Can you work these out from the drawing? Everything is in mm from the part's minimum corner. Round coordinates to 2 decimals unless told otherwise and drop trailing zeros. Loops run counter-clockwise (first coordinate to the right, second up) from the corner with the lowest first, then second, coordinate; pieces in that order, holes last. Notation, with made-up numbers: (71.5, 0.5) -> (120.5, 0.5) arc R30 ccw to (120.5, 22.5) -> close; hole circle Ø8 at (46, 9.25). An arc over 180 degrees is marked (long way). Answer as a JSON object with one key per item and string values.
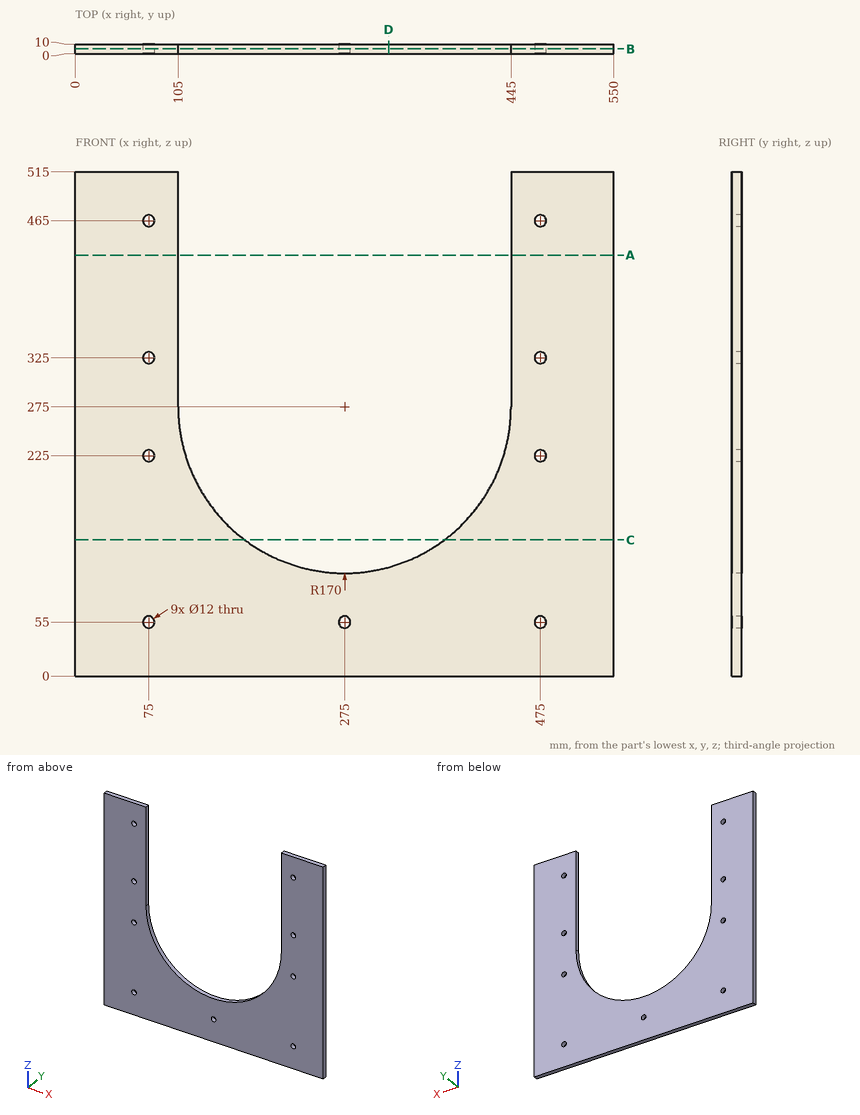
Q1. I want a section at A-A, the plane z = 430. Write out the boundary of the cut face in (x, y), then the cut area to 3 significant figures.
Determined:
{"outline": "(0, 0) -> (105, 0) -> (105, 10) -> (0, 10) -> close; (445, 0) -> (550, 0) -> (550, 10) -> (445, 10) -> close", "area": "2,100 mm²"}
Q2. I want a section at C-C, the plane z = 139. Write out the boundary of the cut face in (x, y).
Determined:
{"outline": "(0, 0) -> (173, 0) -> (173, 10) -> (0, 10) -> close; (377, 0) -> (550, 0) -> (550, 10) -> (377, 10) -> close"}
Q3. I want a section at B-B, the plane y = 5. Give the number of separate pieces and of enclosed holes in the cut face, then the cut area to 3 significant figures.
Determined:
{"separate pieces": "1", "enclosed holes": "9", "area": "155,000 mm²"}
Q4. If I drill on L1, parallel to Z at x = 475, y = 5; L2, parallel to X at y = 5, z = 325; L3, parallel to X at y = 6.75, z = 59, over which ranges is the centre line in solid material (lowest first)? Write a range as [from, to].
Determined:
{"L1": "[0, 49], [61, 219], [231, 319], [331, 459], [471, 515]", "L2": "[0, 69], [81, 105], [445, 469], [481, 550]", "L3": "[0, 70.53], [79.47, 270.53], [279.47, 470.53], [479.47, 550]"}
Q5. I'm going to push flat-ended pins straight in: pin 1 (11 mm diameter, centred on x = 75, z = 325, fed in from -Y); pin 2 (6 mm diameter, centred on x = 263, y = 3, fed in from +Z). Where does each tip first touch, or does it pass through?
Determined:
{"pin 1": "through", "pin 2": "z = 105.66"}
Q6. I want a section at D-D, the plane x = 320. Write out the boundary of the cut face in (y, z).
Determined:
{"outline": "(0, 0) -> (10, 0) -> (10, 111.06) -> (0, 111.06) -> close"}
